Autodesk Inventor part; units mm, degrees
ref_plane "YZ Plane" through (0, 0, 0) normal (1, 0, 0) x (0, 1, 0)
ref_plane "XZ Plane" through (0, 0, 0) normal (0, 1, 0) x (-1, 0, 0)
ref_plane "XY Plane" through (0, 0, 0) normal (0, 0, 1) x (1, 0, 0)
sketch "Esquisse1" plane through (0, 0, 0) normal (0, 0, 1) x (1, 0, 0)
  line L0 (2.0005, 3.465) -> (4.001, 0)
  line L1 (4.001, 0) -> (2.0005, -3.465)
  line L2 (2.0005, -3.465) -> (-2.0005, -3.465)
  line L3 (-2.0005, -3.465) -> (-4.001, 0)
  line L4 (-4.001, 0) -> (-2.0005, 3.465)
  line L5 (-2.0005, 3.465) -> (2.0005, 3.465)
  point P0 (0, 0)
  point P1 (0, 0)
  dimension "d0" = 6.93
extrude "Extrusion1" add sketch "Esquisse1" along normal blind 3
sketch "Esquisse2" plane through (0, 0, 3) normal (0, 0, 1) x (1, 0, 0)
  circle A0 centre (0, 0) radius 3
  dimension "d3" = 6
extrude "Extrusion2" add sketch "Esquisse2" along normal blind 7.5
sketch "Esquisse3" plane through (0, 0, 0) normal (1, 0, 0) x (0, 1, 0)
  line L0 (1.85, 0) -> (0.5, -2)
  line L1 (0.5, -2) -> (0, -2)
  line L2 (0, -2) -> (0, 0)
  line L3 (0, 0) -> (1.85, 0)
  line L4 (0, 0) -> (3.465, 0) construction
  line L5 (0, 0) -> (0, -9.9285)
  dimension "d6" = 2
  dimension "d7" = 1
  dimension "d8" = 3.7
revolve "Révolution1" add sketch "Esquisse3" angle 360 about axis through (0, 0, 0) along (0, 0, -1)
chamfer "Chanfrein1" distance 0.5 angle 45 1 edges at (-3, 0, 10.5)
thread "Filetage1"
sketch "Esquisse4" plane through (0, 0, 0) normal (0, 1, 0) x (-1, 0, 0)
  line L0 (2.0005, 0) -> (4.001, 0)
  line L1 (3.501, 0) -> (4.001, 0.5)
  line L2 (4.001, 0.5) -> (4.001, 0)
  line L3 (4.001, 0) -> (3.501, 0)
  line L4 (0, 0) -> (0, 3.501)
  dimension "d15" = 0.5
  dimension "d16" = 0.5
revolve "Révolution2" cut sketch "Esquisse4" angle 360 about axis through (0, 0, 0) along (0, 0, 1)
fillet "Congé1" radius 0.5 1 edges at (0, -1.85, 0)
sketch "Esquisse5" plane through (0, 0, 10.5) normal (0, 0, 1) x (1, 0, 0)
  point P0 (0, 0)
  point P1 (0, 0)
hole "Perçage1" at (0, 0, 10.5) direction (0, 0, -1) diameter 0.4 end through all counterbore diameter 3.15 counterbore depth 10.5
sketch "Esquisse6" plane through (-2.0005, 3.465, 3) normal (0, 1, 0) x (1, 0, 0)
  line L0 (1.4995, 3) -> (2.5016, 3) construction
  line L1 (4.7508, 3) -> (2.5016, 3) construction
  line L2 (6.0016, 0) -> (4.001, 0) construction
  point P0 (2.0005, 3)
  point P1 (2.0005, 1.5)
  point P2 (4.001, 1.5)
  point P3 (2.0005, 3)
  dimension "d26" = 3
  dimension "d27" = 1.5
hole "Perçage2" at (0, 3.465, 1.5) direction (0, -1, 0) diameter 1 depth 0.01 tip angle 118
pattern_circular "Réseau circulaire1" count 2 over 60 about axis through (0, 0, -5.8801) along (0, 0, 1) of "Perçage2"
chamfer "Chanfrein2" distance 1.375 angle 45 1 edges at (0, 1.575, 0)
equation "\"d16\" = d15"
properties part number "Buse 04" material "Laiton, jaune doux"
Here's how the part is built. I have some questions about the finished solid (model axes, mm). A direction names the side the tool comes from. Coordinates: 2 decimals unless noted, no trailing zeros. Loops run counter-clockwise (first coordinate to the right, second up) from the corner with the lowest first, then second, coordinate; pieces in that order, holes last.
1. I need wall thicknesses on L1, parallel to Y at x = 0, z = 5 (3 decimals); L2, parallel to Z at x = -0.25, y = 2.25; L3, parallel to Z at x = 2.5, y = 2.25. Which ranges of each line are inside material? Lowest first, please.
2. For P1, Ø2, axis at x = -1.5, y = -0.5, coming from the -Z side; P2, Ø1, axis at x = -1.5, y = -1.5, coming from the -Z side; P3, Ø1, axis at x = -2, y = 2.5, coming from the -Z side, each with a flat end and sliding along its axis, tell me the tip position at first contact or that it passes through.
3. If we mould it in two halves opening along X, with no side actions, what happens to faces 4 (the flat face through (3, 1, 3)), 5 (the conical face through (-1.805, 3.165, 0.142)), 6 (the cylindrical face through (0.96, 1.25, 5.87))? For each: pulls with the +X half, pulls with the -X half, needs draft (parallel to the pull), parting line crosses it, or undercut.
4. Imagine slicing it at A-A, the plane z = 0.75. Please give me the cut outline in (x, y) (1 decimal).
5. Imagine slicing it at B-B, the plane z = 8.5. Please give me the cut outline in (x, y) (3 decimals).
6. For faces 1 (the flat face through (2, 2, 0)), 2 (the flat face through (2.987, 1.757, 1.479)), 3 (the cylindrical face through (-3, 0, 6)), which set-ups out of +Z, -Z, +X, -X, +Y, -Y let a thin tool reach every point of the face, with its end or its side?
Taken from the geometry:
1. L1: y = -3 to -1.575, 1.575 to 3
1. L2: z = 0 to 10.5
1. L3: z = 0 to 3
2. P1: stops at z = -1.88
2. P2: stops at z = -0.34
2. P3: stops at z = 0
3. face 4: needs draft
3. face 5: pulls with the -X half
3. face 6: undercut
4. outline: (-4, 0) - (-2, -3.5) - (2, -3.5) - (4, 0) - (2, 3.5) - (-2, 3.5) - close; hole circle Ø1.9 at (0, 0)
5. outline: circle Ø6 at (0, 0); hole circle Ø3.15 at (0, 0)
6. face 1: -Z
6. face 2: +Z, -Z, +X, +Y
6. face 3: +Z
